```python
from build123d import *

# Parameters (mm, degrees)
F0_R     = 11.049
F1_DEPTH = 6.35


with BuildPart() as f1:
    # F0 (on Top) → F1 (new body)
    with BuildSketch(Plane.XY):
        with BuildLine():
            ThreePointArc((-11.3469625039, 20.0920200438), (-14.4854082565, 4.9914875059), (-26.2741162088, -4.9534755149))
            ThreePointArc((-26.2741162088, -4.9534755149), (-16.5077935225, -8.934489521), (-12.3076651672, -18.6086020451))
            ThreePointArc((-12.3076651672, -18.6086020451), (0.649772882, -14.1418626943), (13.4943491716, -18.9234755149))
            ThreePointArc((13.4943491716, -18.9234755149), (17.3328597235, -8.6100846058), (27.4479022012, -4.2757898563))
            ThreePointArc((27.4479022012, -4.2757898563), (15.2201160848, 5.4859259906), (11.7737009685, 20.7480383092))
            ThreePointArc((11.7737009685, 20.7480383092), (6.7498223767, 15.9073674809), (0, 14.1434661071))
            ThreePointArc((0, 14.1434661071), (-6.4058342939, 15.720767845), (-11.3469625039, 20.0920200438))
        make_face()
        with BuildLine():
            ThreePointArc((13.97, 0), (-9.8782817332, -9.8782817332), (0, 13.97))
            ThreePointArc((0, 13.97), (9.8782817332, 9.8782817332), (13.97, 0))
        make_face(mode=Mode.SUBTRACT)
        with BuildLine():
            ThreePointArc((13.97, 0), (9.8782817332, 9.8782817332), (0, 13.97))
            ThreePointArc((0, 13.97), (-9.8782817332, -9.8782817332), (13.97, 0))
        make_face()
        with BuildLine():
            ThreePointArc((11.6814433874, 0), (-8.2600278333, -8.2600278333), (0, 11.6814433874))
            ThreePointArc((0, 11.6814433874), (8.2600278333, 8.2600278333), (11.6814433874, 0))
        make_face(mode=Mode.SUBTRACT)
        with BuildLine():
            ThreePointArc((-26.2741162088, -4.9534755149), (-36.1348230129, -9.0276500657), (-40.2440279254, -18.8738103292))
            ThreePointArc((-40.2440279254, -18.8738103292), (-36.068722537, -25.9778704776), (-30.6538718182, -32.1891696469))
            ThreePointArc((-30.6538718182, -32.1891696469), (-18.0895052181, -30.2448289204), (-12.3041162088, -18.9234755149))
            ThreePointArc((-12.3041162088, -18.9234755149), (-12.3050034765, -18.7660287802), (-12.3076651672, -18.6086020451))
            ThreePointArc((-12.3076651672, -18.6086020451), (-16.5077935225, -8.934489521), (-26.2741162088, -4.9534755149))
        make_face()
        with Locations((-26.2741162088, -18.9234755149)):
            Circle(F0_R, mode=Mode.SUBTRACT)
        with BuildLine():
            ThreePointArc((-13.7965338929, 27.94), (-12.227697713, 24.1233976847), (-11.3469625039, 20.0920200438))
            ThreePointArc((-11.3469625039, 20.0920200438), (-6.4058342939, 15.720767845), (0, 14.1434661071))
            ThreePointArc((0, 14.1434661071), (6.7498223767, 15.9073674809), (11.7737009685, 20.7480383092))
            ThreePointArc((11.7737009685, 20.7480383092), (12.4990400343, 24.4244821494), (13.7965338929, 27.94))
            ThreePointArc((13.7965338929, 27.94), (0, 41.7365338929), (-13.7965338929, 27.94))
        make_face()
        with BuildLine():
            ThreePointArc((11.049, 27.94), (7.8128228253, 20.1271771747), (0, 16.891))
            ThreePointArc((0, 16.891), (-7.8128228253, 35.7528228253), (11.049, 27.94))
        make_face(mode=Mode.SUBTRACT)
        with BuildLine():
            ThreePointArc((31.1400760327, -31.7190505009), (37.0174753812, -24.6070928067), (41.3000458498, -16.4349844175))
            ThreePointArc((41.3000458498, -16.4349844175), (36.6637566928, -7.7467934285), (27.4479022012, -4.2757898563))
            ThreePointArc((27.4479022012, -4.2757898563), (17.3328597235, -8.6100846058), (13.4943491716, -18.9234755149))
            ThreePointArc((13.4943491716, -18.9234755149), (19.2469473442, -29.5553097149), (31.1400760327, -31.7190505009))
        make_face()
        with Locations((27.4479022012, -18.2457898563)):
            Circle(F0_R, mode=Mode.SUBTRACT)
        with BuildLine():
            ThreePointArc((41.4179022012, -18.2457898563), (41.3884069763, -17.338471492), (41.3000458498, -16.4349844175))
            ThreePointArc((41.3000458498, -16.4349844175), (37.0174753812, -24.6070928067), (31.1400760327, -31.7190505009))
            ThreePointArc((31.1400760327, -31.7190505009), (38.5551198642, -26.7187241642), (41.4179022012, -18.2457898563))
        make_face()
        with BuildLine():
            ThreePointArc((-30.6538718182, -32.1891696469), (-36.068722537, -25.9778704776), (-40.2440279254, -18.8738103292))
            ThreePointArc((-40.2440279254, -18.8738103292), (-37.6100004347, -27.0879490936), (-30.6538718182, -32.1891696469))
        make_face()
    extrude(amount=F1_DEPTH)


solid = f1.part
```
Read the model definition and answer for the solid it produces. Units are mm, in the model's axes. Round coordinates to 2 decimals unless told otherwise and drop trailing zeros. Write each loop counter-clockwise with the first axis right and the second up, starting at its lowest first coordinate (ties: lowest second). Pieces come first, ordered by that corner, then holes. Notation, with made-up numbers: M -2,56.5 L 35,56.5 A20 ccw 35,75.5 Z; hole C 78.25,37.5 d5. An arc over 180 degrees is marked long. One line per item, written item: value.
Q1. For a pull along Y with two mould halves and no side action, classify faces 1 (the cylindrical face through (-15.735, -15.605, 3.131)), 2 (the cylindrical face through (0.303, 41.733, 3.131)), 3 (the flat face through (-3, -12, 6.35)) as +Y half, -Y half, draft (parallel to the pull), parting line (faces both ways), or undercut.
Data:
face 1: undercut
face 2: +Y half
face 3: draft
Q2. Straight lines are drawn through the part: line 1 (Y direction, x = 8.5, z = 1.75); line 2 (Y direction, x = -10, z = 6); line 3 (X direction, y = -25, z = 3). For each, find the intervals that lie inside material, in ascending order. Write a range as [from, to].
Data:
line 1: [-15.82, -8.01], [8.01, 20.88], [35, 38.81]
line 2: [-17.01, -6.04], [6.04, 23.24], [32.64, 37.44]
line 3: [-38.85, -35.5], [-17.05, -13.69], [15.22, 18.7], [36.19, 39.68]
Q3. Find section D-D on x = 21. Write down the section's boundary in (y, z), plus the area to 3 significant figures.
Data:
outline: M -30.64,0 L -27.22,0 L -27.22,6.35 L -30.64,6.35 Z; M -9.27,0 L -0.82,0 L -0.82,6.35 L -9.27,6.35 Z
area: 75.4 mm2
Q4. Find section B-B on y = 1.5. Write down the section's boundary in (x, z).
Data:
outline: M -17.03,0 L -11.58,0 L -11.58,6.35 L -17.03,6.35 Z; M 11.58,0 L 18.36,0 L 18.36,6.35 L 11.58,6.35 Z
Q5. Find section C-C on x = -2. Write down the section's boundary in (y, z).
Data:
outline: M -14.28,0 L -11.51,0 L -11.51,6.35 L -14.28,6.35 Z; M 11.51,0 L 17.07,0 L 17.07,6.35 L 11.51,6.35 Z; M 38.81,0 L 41.59,0 L 41.59,6.35 L 38.81,6.35 Z
Q6. Find section A-A on z = 1. Write down the section's boundary in (x, y), plus the area to 3 significant figures.
Data:
outline: M -26.27,-4.95 A13.97 ccw long -12.3,-18.92 A13.97 ccw -12.31,-18.61 A20.31 cw 13.49,-18.92 A13.97 ccw long 27.45,-4.28 A23.63 cw 13.8,27.94 A13.8 ccw -13.8,27.94 A23.62 cw Z; hole C -26.27,-18.92 d22.1; hole C 0,0 d23.36; hole C 0,27.94 d22.1; hole C 27.45,-18.25 d22.1
area: 1,260 mm2
Q7. Flat-ended cylindrical pins translate along their axes: pin 1 Ø2 at (y, z) = (34, 3) entering from -X; pin 2 Ø2 at (x, z) = (24, 4.5) entering from -Y; pin 3 Ø17.5 at (x, y) = (-26.27, -18.92) entering from +Z; pin 4 Ø2 at (x, z) = (33, 3.5) entering from -Y. Find the tip coordinate at first contact, or state that the pin passes through.
Data:
pin 1: x = -12.84
pin 2: y = -32
pin 3: through
pin 4: y = -31.45
